Can you work these out from the drawing? Everything is in mm from the part's minimum corner. Round coordinates to 2 decimals unless told otherwise and drop trailing zeros. Write each loop counter-clockwise with the first axis right and the second up, starting at its lowest first coordinate (ties: lowest second). Pieces come first, ordered by that corner, then holes. Notation, with made-up numbers: M -26,83 L 7,83 A15 ccw 7,100 Z; hole C 33.25,69 d11. An arc over 180 degrees is marked long. Use one line per item in the form item = value. Start each with the question number.
Q1. I want a section at C-C on y = 95.25. List the corners of the cut face in (x, z) for me (3 decimals), and give its area (3 significant figures).
Q2. I want a section at D-D on z = 1.1. State how many separate pieces and enclosed holes the cut face has, and give its area (3 significant figures).
Q3. I want a section at A-A on y = 57.15. List the corners of the cut face in (x, z) for me (3 decimals).
Q4. I need wall thicknesses on line 1 along X through (y, z) = (95.25, 0.85); line 2 along Y through (x, z) = (6.35, 1.65); line 3 along X through (y, z) = (44.45, 2.25). Which ranges of each line are inside material? Lowest first, please. Write a range as from..to.
Q5. I want a section at B-B on x = 69.85. List the corners of the cut face in (y, z) for me (3 decimals).
Q6. I'm going to push a flat-ended pin straight in: pin 1 Ø1.6 at (x, z) = (44, 2) entering from -Y. Where does the tip first touch, or does it pass through?
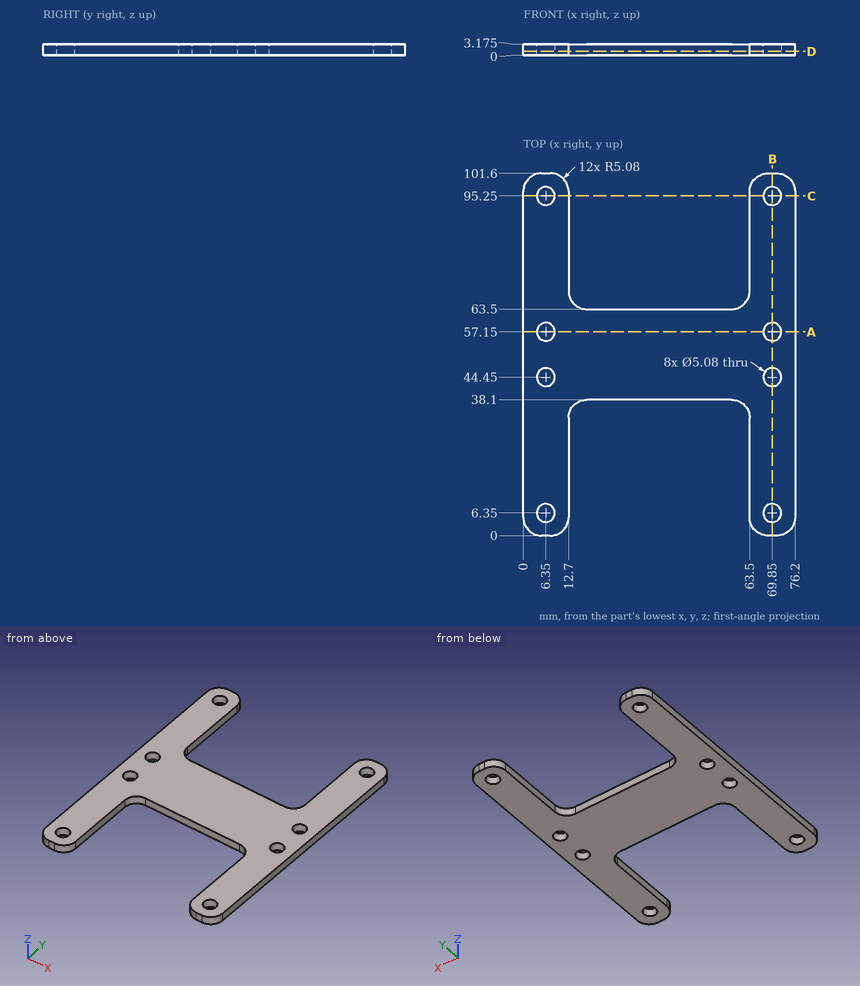
Reported:
q1.outline = M 0,0 L 3.81,0 L 3.81,3.175 L 0,3.175 Z; M 8.89,0 L 12.7,0 L 12.7,3.175 L 8.89,3.175 Z; M 63.5,0 L 67.31,0 L 67.31,3.175 L 63.5,3.175 Z; M 72.39,0 L 76.2,0 L 76.2,3.175 L 72.39,3.175 Z
q1.area = 48.4 mm^2
q2.separate_pieces = 1
q2.enclosed_holes = 8
q2.area = 3,690 mm^2
q3.outline = M 0,0 L 3.81,0 L 3.81,3.175 L 0,3.175 Z; M 8.89,0 L 67.31,0 L 67.31,3.175 L 8.89,3.175 Z; M 72.39,0 L 76.2,0 L 76.2,3.175 L 72.39,3.175 Z
q4.line_1 = 0..3.81, 8.89..12.7, 63.5..67.31, 72.39..76.2
q4.line_2 = 0..3.81, 8.89..41.91, 46.99..54.61, 59.69..92.71, 97.79..101.6
q4.line_3 = 0..3.81, 8.89..67.31, 72.39..76.2
q5.outline = M 0,0 L 3.81,0 L 3.81,3.175 L 0,3.175 Z; M 8.89,0 L 41.91,0 L 41.91,3.175 L 8.89,3.175 Z; M 46.99,0 L 54.61,0 L 54.61,3.175 L 46.99,3.175 Z; M 59.69,0 L 92.71,0 L 92.71,3.175 L 59.69,3.175 Z; M 97.79,0 L 101.6,0 L 101.6,3.175 L 97.79,3.175 Z
q6.pin_1 = 38.1
